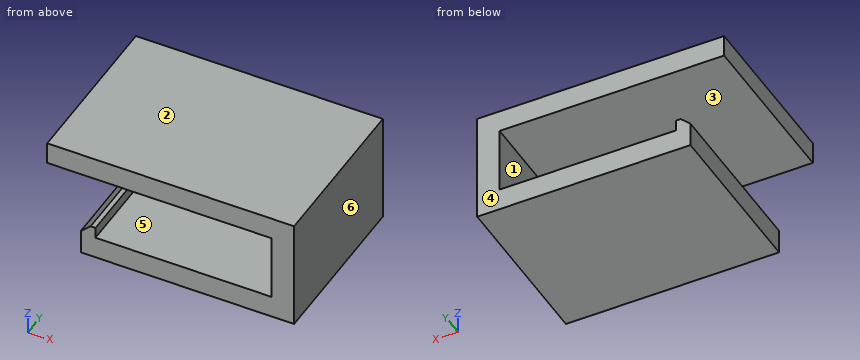
from build123d import *

# Parameters (mm, degrees)
F0_W     = 19
F0_H     = 15
F1_DEPTH = 2
F2_W     = 2
F2_H     = 15
F3_DEPTH = 8
F4_W     = 15
F4_H     = 2
F5_DEPTH = 20
F6_W     = 1.3
F6_H     = 15
F7_DEPTH = 1
F9_DEPTH = 25


with BuildPart() as f1:
    # F0 (on Top) → F1 (new body)
    with BuildSketch(Plane.XY):
        Rectangle(F0_W, F0_H)
    extrude(amount=F1_DEPTH)

    # F2 (on face) → F3 (join)
    with BuildSketch(Plane.XY.offset(2)):
        with Locations((8.5, 0)):
            Rectangle(F2_W, F2_H)
    extrude(amount=F3_DEPTH)

    # F4 (on face) → F5 (join)
    with BuildSketch(Plane(origin=(7.5, 0, 0), x_dir=(0, -1, 0), z_dir=(-1, 0, 0))):
        with Locations((0, 9)):
            Rectangle(F4_W, F4_H)
    extrude(amount=F5_DEPTH)

    # F6 (on face) → F7 (join)
    with BuildSketch(Plane.XY.offset(2)):
        with Locations((-8.85, 0)):
            Rectangle(F6_W, F6_H)
    extrude(amount=F7_DEPTH)

    # F8 (on face) → F9 (cut)
    with BuildSketch(Plane.XZ.offset(7.5)):
        Polygon((-9.5, 3), (-9.5, 2.195644), (-8.629206, 3), align=None)
    extrude(amount=-F9_DEPTH, mode=Mode.SUBTRACT)


solid = f1.part
The listing builds one solid part. Answer for the finished solid, in the listing's coordinates (mm). Face numbers are marked on the shaded views. A direction names the side the tool comes from. Coordinates: 2 decimals unless noted, no trailing zeros. Order: outer loops, then holes, each group sorted by start corner. A loop starts at its lowest first (then second) coordinate and runs counter-clockwise, first axis right, second up.
Q1. A cutting plane is placed at D-D, the plane z = 7.5. Write down the section's boundary in (x, y).
Q2. Given P1, Ø1.8, axis at y = 2.5, z = 4.5, coming from the -X side; P2, Ø1.8, axis at y = 3, z = 1, coming from the -X side, each flat-ended and moving along its own axis, determine where each tip first touches the part or whether it passes through.
Q3. For a pull along X with two mould halves and no side action, classify the marked faces 4, 5 and 6 as pulls with the +X half, pulls with the -X half, needs draft (parallel to the pull), parting line crosses it, or undercut.
Q4. A cutting plane is placed at B-B, the plane z = 2.75. Write down the section's boundary in (x, y).
Q5. Consider line 1 (Z direction, x = -1.75, y = 4); line 2 (X direction, y = -5, z = 7.75); line 3 (Z direction, x = -10.5, y = 5.75). Determine where each line is inside the solid, lowest interval first.
Q6. Which of the six approach directions +Z, -Z, +X, -X, +Y, -Y give full straight-line access (tool end or side, diameter ignored) to the marked faces 1, 2 and 3?
Q7. A cutting plane is placed at A-A, the plane x = 3.25. Write down the section's boundary in (y, z).
Q8. A cutting plane is placed at C-C, the plane y = 3.5. Write down the section's boundary in (x, z), and give its area (4 significant figures).
Answers follow:
1. outline: (7.5, -7.5) - (9.5, -7.5) - (9.5, 7.5) - (7.5, 7.5) - close
2. P1: stops at x = 7.5
2. P2: stops at x = -9.5
3. face 4: needs draft
3. face 5: undercut
3. face 6: pulls with the +X half
4. outline: (-8.9, -7.5) - (-8.2, -7.5) - (-8.2, 7.5) - (-8.9, 7.5) - close; (7.5, -7.5) - (9.5, -7.5) - (9.5, 7.5) - (7.5, 7.5) - close
5. line 1: z = 0 to 2, 8 to 10
5. line 2: x = 7.5 to 9.5
5. line 3: z = 8 to 10
6. face 1: +Y, -Y
6. face 2: +Z, +X, -X, +Y, -Y
6. face 3: -X, +Y, -Y
7. outline: (-7.5, 0) - (7.5, 0) - (7.5, 2) - (-7.5, 2) - close; (-7.5, 8) - (7.5, 8) - (7.5, 10) - (-7.5, 10) - close
8. outline: (-12.5, 8) - (7.5, 8) - (7.5, 2) - (-8.2, 2) - (-8.2, 3) - (-8.63, 3) - (-9.5, 2.2) - (-9.5, 0) - (9.5, 0) - (9.5, 10) - (-12.5, 10) - close
8. area: 94.95 mm2
